Source: CAD feature listing. Evaluate the final solid. Frame: model axes, mm. A direction names the side the tool comes from. Round coordinates to 2 decimals unless told otherwise and drop trailing zeros. Write each loop counter-clockwise with the first axis right and the second up, starting at its lowest first coordinate (ties: lowest second). Pieces come first, ordered by that corner, then holes.
from build123d import *

# Parameters (mm, degrees)
F1_DEPTH = 2


with BuildPart() as f1:
    # F0 (on Top) → F1 (new body, symmetric)
    with BuildSketch(Plane.XY):
        Polygon((170, 85), (-170, 85), (-170, -85), align=None)
        Polygon((-145, -44.5491502813), (-145, 60), (64.0983005625, 60), align=None, mode=Mode.SUBTRACT)
    extrude(amount=F1_DEPTH, both=True)


solid = f1.part
1) Section query C-C on y = 45.5. Return the cut outline in (x, z), then the cut area to 3 significant figures.
Taken from the geometry:
outline: (-170, -2) - (-145, -2) - (-145, 2) - (-170, 2) - close; (35.1, -2) - (91, -2) - (91, 2) - (35.1, 2) - close
area: 324 mm2
2) Section query A-A on x = -76.5. Return the cut outline in (y, z).
Taken from the geometry:
outline: (-38.25, -2) - (-10.3, -2) - (-10.3, 2) - (-38.25, 2) - close; (60, -2) - (85, -2) - (85, 2) - (60, 2) - close
3) Section query D-D on x = 82. Return the cut outline in (y, z), then the cut area to 3 significant figures.
Taken from the geometry:
outline: (41, -2) - (85, -2) - (85, 2) - (41, 2) - close
area: 176 mm2
4) Material intervals for line 1 (X direction, y = -29, z = 1.5); line 2 (X direction, y = 36.5, z = 0.3); line 3 (Y direction, x = -89.5, z = 0.5), sorted ascending.
Taken from the geometry:
line 1: x = -170 to -145, -113.9 to -58
line 2: x = -170 to -145, 17.1 to 73
line 3: y = -44.75 to -16.8, 60 to 85
5) Section query B-B on z = -0.7. Return the cut outline in (x, y), then the cut area to 3 significant figures.
Taken from the geometry:
outline: (-170, -85) - (170, 85) - (-170, 85) - close; hole (-145, -44.55) - (64.1, 60) - (-145, 60) - close
area: 18,000 mm2
6) Reachability of faces 1 (the face through (-2, -1, 0)), 2 (the face through (-38.987, 8.457, 0.028)) from +Z, -Z, +X, -X, +Y, -Y: full face, straight path, thin tool, end or side. Return the list, or none.
Taken from the geometry:
face 1: +Z, -Z, +X, -Y
face 2: +Z, -Z
